from build123d import *

# Parameters (mm, degrees)
SKETCH1_R           = 1.6
SKETCH1_R_2         = 18.5
SKETCH1_R_3         = 14.2875
SKETCH1_W           = 9.525
SKETCH1_H           = 76.2
BOSS_EXTRUDE1_DEPTH = 3
CUT_EXTRUDE1_DEPTH  = 109.338539954
CIRPATTERN1_COUNT   = 3


with BuildPart() as part:
    # Sketch1 → Boss-Extrude1 (new body)
    # profile 1 of 2: a face of its own
    with BuildSketch(Plane(origin=(0, 0, 0), x_dir=(0, 0, -1), z_dir=(1, 0, 0))):
        with BuildLine():
            ThreePointArc((4.931768052, -55.34319353), (-7.747067981, -55.019763212), (-20.022244586, -51.829539145))
            Line((-20.022244586, -51.829539145), (-55.5625, -38.1))
            Line((-55.5625, -38.1), (-55.5625, 38.1))
            Line((-55.5625, 38.1), (-20.022244586, 51.829539145))
            ThreePointArc((-20.022244586, 51.829539145), (-7.747067981, 55.019763212), (4.931768052, 55.34319353))
            Line((4.931768052, 55.34319353), (70.31294072, 49.516916477))
            ThreePointArc((70.31294072, 49.516916477), (86.442097474, 41.538651245), (92.957236583, 24.765))
            Line((92.957236583, 24.765), (92.957236583, -24.765))
            ThreePointArc((92.957236583, -24.765), (86.442097474, -41.538651245), (70.31294072, -49.516916477))
            Line((70.31294072, -49.516916477), (4.931768052, -55.34319353))
        make_face()
        with Locations((-50.8, 0)):
            Circle(SKETCH1_R, mode=Mode.SUBTRACT)
        with Locations((0, -50.8)):
            Circle(SKETCH1_R, mode=Mode.SUBTRACT)
        with Locations((50.8, 0)):
            Circle(SKETCH1_R, mode=Mode.SUBTRACT)
        with Locations((0, 50.8)):
            Circle(SKETCH1_R, mode=Mode.SUBTRACT)
        Circle(SKETCH1_R_2, mode=Mode.SUBTRACT)
        with Locations((68.107236583, -24.765)):
            Circle(SKETCH1_R_3, mode=Mode.SUBTRACT)
        with Locations((68.107236583, 24.765)):
            Circle(SKETCH1_R_2, mode=Mode.SUBTRACT)
    # profile 2 of 2: a face of its own
    with BuildSketch(Plane(origin=(0, 0, 0), x_dir=(0, 0, -1), z_dir=(1, 0, 0))):
        with Locations((-60.325, 0)):
            Rectangle(SKETCH1_W, SKETCH1_H)
    extrude(amount=BOSS_EXTRUDE1_DEPTH)

    # Sketch2 → Cut-Extrude1 (cut, symmetric)
    with BuildSketch(Plane.ZY):
        with BuildLine():
            ThreePointArc((-86.182075073, 32.962919695), (-88.406895893, 32.146316407), (-87.226207177, 30.09140941))
            ThreePointArc((-87.226207177, 30.09140941), (-86.398498104, 29.550435617), (-86.209643196, 28.579823038))
            ThreePointArc((-86.209643196, 28.579823038), (-85.493518863, 31.086960811), (-84.432027328, 33.46851694))
            ThreePointArc((-84.432027328, 33.46851694), (-85.200208842, 32.845899791), (-86.182075073, 32.962919695))
        make_face()
    cut_extrude1 = extrude(amount=CUT_EXTRUDE1_DEPTH, both=True, mode=Mode.SUBTRACT)

    # CirPattern1: Cut-Extrude1 ×3 about axis
    cirpattern1_axis = Axis((0, 24.765, -68.107236583), (1, 0, 0))
    for i in range(1, CIRPATTERN1_COUNT):
        add(cut_extrude1.rotate(cirpattern1_axis, i * 360 / CIRPATTERN1_COUNT), mode=Mode.SUBTRACT)


solid = part.part
For this review, take the finished solid that the model builds, in its own axes (mm). A direction names the side the tool comes from. Give positions to 0.01 mm unless a question says otherwise; leave off trailing zeros. Loops run counter-clockwise (first coordinate to the right, second up) from the corner with the lowest first, then second, coordinate; pieces in that order, holes last. Notation, with made-up numbers: (-29, 56.25) - (26, 56.25) arc R16 ccw to (26, 87.25) - close; hole circle Ø8 at (73.25, 89). An arc over 180 degrees is marked (long way). Write each question's results on one line, items separated by ' | '.
(1) For pin 1 Ø22 at (y, z) = (0, 0) entering from +X; pin 2 Ø4 at (y, z) = (0, 50.8) entering from +X, all flat-tipped, find the tip position at first contact; note any pin that passes through.
Conclusion:
pin 1: through | pin 2: x = 3
(2) Take a section at D-D (x = 1.8). State how many separate pieces and enclosed holes the cut face has, then the cut area to 3 significant figures.
Conclusion:
separate pieces: 1 | enclosed holes: 7 | area: 12,600 mm^2
(3) For line 1 along Y through (x, z) = (2.3, 0); line 2 along Z through (x, y) = (2.6, -25.5); line 3 along Z through (x, y) = (0.85, -14), list the stretches that pass through material, from the lowest coordinate up.
Conclusion:
line 1: -55.56 to -52.4, -49.2 to -18.5, 18.5 to 49.2, 52.4 to 55.56 | line 2: -92.95 to -82.38, -53.84 to 65.09 | line 3: -92.96 to -77.5, -58.71 to -12.09, 12.09 to 65.09
(4) Draft analysis for pull direction Z (two halves, no side actions). For faces 1 (the cylindrical face through (1.479, -55.044, 7.571)), 2 (the cylindrical face through (1.48, -18.06, 4.01)), 3 (the flat face through (1.48, 52.47, -37.16)), 4 (the cylindrical face through (1.479, -15.109, -57.577)), state which applies: +Z half, -Z half, draft (parallel to the pull), parting line (faces both ways), or undercut.
Conclusion:
face 1: parting line | face 2: undercut | face 3: -Z half | face 4: undercut
(5) For faces 5 (the cylindrical face through (1.479, 41.728, -86.267)), 6 (the flat face through (1, 38.1, 60)), 7 (the cylindrical face through (1.48, 42.94, -71.56)), list the 3-axis set-ups (+Z, -Z, +X, -X, +Y, -Y) from which the entire face can be reached by the end or side of a thin tool; tool diameter is ignored.
Conclusion:
face 5: -Z, +X, -X, +Y | face 6: +Z, +X, -X, +Y | face 7: +X, -X
(6) Take a section at C-C (z = -57.5). Give the boundary of the cut face in (x, y).
Conclusion:
outline: (0, -50.66) - (3, -50.66) - (3, -34.34) - (0, -34.34) - close; (0, -15.19) - (3, -15.19) - (3, 9.61) - (0, 9.61) - close; (0, 39.92) - (3, 39.92) - (3, 50.66) - (0, 50.66) - close
(7) Take a section at A-A (y = 0). Give the boundary of the cut face in (x, z).
Conclusion:
outline: (0, -92.96) - (3, -92.96) - (3, -52.4) - (0, -52.4) - close; (0, -49.2) - (3, -49.2) - (3, -18.5) - (0, -18.5) - close; (0, 18.5) - (3, 18.5) - (3, 49.2) - (0, 49.2) - close; (0, 52.4) - (3, 52.4) - (3, 65.09) - (0, 65.09) - close
(8) Take a section at B-B (z = 50.8). Give the boundary of the cut face in (x, y).
Conclusion:
outline: (0, -39.94) - (3, -39.94) - (3, -1.6) - (0, -1.6) - close; (0, 1.6) - (3, 1.6) - (3, 39.94) - (0, 39.94) - close
